The model under review builds one solid part; all positions refer to its coordinate system, in mm. A direction names the side the tool comes from. Round coordinates to 2 decimals unless told otherwise and drop trailing zeros. Write each loop counter-clockwise with the first axis right and the second up, starting at its lowest first coordinate (ties: lowest second). Pieces come first, ordered by that corner, then holes. Notation, with made-up numbers: (3, 15.5) - (27, 15.5) arc R7 ccw to (27, 21.5) - close; hole circle Ø5 at (76.5, 86). An arc over 180 degrees is marked (long way). One line per question, with ' | ' between items. Start each with the question number.
```python
from build123d import *

# Parameters (mm, degrees)
SKETCH1_W           = 183
SKETCH1_H           = 80.5
SKETCH1_W_2         = 163
SKETCH1_H_2         = 23
SKETCH1_R           = 1.6
BOSS_EXTRUDE1_DEPTH = 3.2
SKETCH1_3_W         = 183
SKETCH1_3_H         = 80.5
SKETCH1_3_R         = 1.6
SKETCH1_3_W_2       = 163
SKETCH1_3_H_2       = 23
BOSS_EXTRUDE2_DEPTH = 3


with BuildPart() as part:
    # Sketch1 → Boss-Extrude1 (new body)
    with BuildSketch(Plane(origin=(0, 0, 0), x_dir=(1, 0, 0), z_dir=(0, 1, 0))):
        Rectangle(SKETCH1_W, SKETCH1_H)
        with Locations((0, 17.25)):
            Rectangle(SKETCH1_W_2, SKETCH1_H_2, mode=Mode.SUBTRACT)
        Polygon((83.5, 2.75), (83.5, -2.75), (81.5, -2.75), (-81.5, -2.75), (-83.5, -2.75), (-83.5, 2.75), align=None, mode=Mode.SUBTRACT)
        with Locations((0, -17.25)):
            Rectangle(SKETCH1_W_2, SKETCH1_H_2, mode=Mode.SUBTRACT)
        Polygon((83.5, -31.75), (83.5, -37.25), (-81.5, -37.25), (-83.5, -37.25), (-83.5, -31.75), align=None, mode=Mode.SUBTRACT)
        Polygon((81.5, 37.25), (83.5, 37.25), (83.5, 31.75), (-83.5, 31.75), (-83.5, 37.25), align=None, mode=Mode.SUBTRACT)
        with Locations((-87.5, -34.5)):
            Circle(SKETCH1_R, mode=Mode.SUBTRACT)
        with Locations((-87.5, 0)):
            Circle(SKETCH1_R, mode=Mode.SUBTRACT)
        with Locations((-87.5, 34.5)):
            Circle(SKETCH1_R, mode=Mode.SUBTRACT)
        with Locations((87.5, 34.5)):
            Circle(SKETCH1_R, mode=Mode.SUBTRACT)
        with Locations((87.5, -34.5)):
            Circle(SKETCH1_R, mode=Mode.SUBTRACT)
        with Locations((87.5, 0)):
            Circle(SKETCH1_R, mode=Mode.SUBTRACT)
    extrude(amount=BOSS_EXTRUDE1_DEPTH)

    # Sketch1<3> → Boss-Extrude2 (add)
    with BuildSketch(Plane(origin=(0, 0, 0), x_dir=(1, 0, 0), z_dir=(0, 1, 0))):
        Rectangle(SKETCH1_3_W, SKETCH1_3_H)
        with Locations((-87.5, -34.5)):
            Circle(SKETCH1_3_R, mode=Mode.SUBTRACT)
        with Locations((0, -17.25)):
            Rectangle(SKETCH1_3_W_2, SKETCH1_3_H_2, mode=Mode.SUBTRACT)
        with Locations((87.5, -34.5)):
            Circle(SKETCH1_3_R, mode=Mode.SUBTRACT)
        with Locations((-87.5, 0)):
            Circle(SKETCH1_3_R, mode=Mode.SUBTRACT)
        with Locations((0, 17.25)):
            Rectangle(SKETCH1_3_W_2, SKETCH1_3_H_2, mode=Mode.SUBTRACT)
        with Locations((-87.5, 34.5)):
            Circle(SKETCH1_3_R, mode=Mode.SUBTRACT)
        with Locations((87.5, 0)):
            Circle(SKETCH1_3_R, mode=Mode.SUBTRACT)
        with Locations((87.5, 34.5)):
            Circle(SKETCH1_3_R, mode=Mode.SUBTRACT)
    extrude(amount=-BOSS_EXTRUDE2_DEPTH)


solid = part.part
```
1. Machinability: for faces 3 (the face through (-1, 0, 40.25)), 4 (the face through (-81.5, 0, 17)), 5 (the face through (83.5, 2, -35)), which of the approach directions +Z, -Z, +X, -X, +Y, -Y give a long, thin tool a straight path to every point of the face, cutting with its end or side? Answer none if there is none.
2. Add section A-A, the plane z = 20. Write out the cut boundary in (x, y), then the cut area to 3 significant figures.
3. Add section C-C, the plane x = 8. Write out the cut boundary in (y, z), then the cut area to 3 significant figures.
4. The part is to be moulded in two halves that separate along X. For faces 1 (the face through (-22, -3, -1)), 2 (the face through (-1, 0, -5.75)), say which applies: pulls with the +X half, pulls with the -X half, needs draft (parallel to the pull), parting line crosses it, or undercut.
5. Wall thickness on line 1 along Z through (x, y) = (-87.5, -0.75); line 2 along X through (y, z) = (0.5, 0); line 3 along Z through (x, y) = (-42.5, 0.5): over which ranges is each line inside the solid? List them lowest first. Write a range as [from, to].
6. Add section B-B, the plane y = -1.75. State how many separate pieces and enclosed holes the cut face has, then the cut area to 3 significant figures.
Geometry check:
1) face 3: +Z, +X, -X, +Y, -Y | face 4: +Y, -Y | face 5: +Y
2) outline: (-91.5, -3) - (-81.5, -3) - (-81.5, 3.2) - (-91.5, 3.2) - close; (81.5, -3) - (91.5, -3) - (91.5, 3.2) - (81.5, 3.2) - close | area: 124 mm2
3) outline: (-3, -40.25) - (3.2, -40.25) - (3.2, -37.25) - (0, -37.25) - (0, -31.75) - (3.2, -31.75) - (3.2, -28.75) - (-3, -28.75) - close; (-3, -5.75) - (3.2, -5.75) - (3.2, -2.75) - (0, -2.75) - (0, 2.75) - (3.2, 2.75) - (3.2, 5.75) - (-3, 5.75) - close; (-3, 28.75) - (3.2, 28.75) - (3.2, 31.75) - (0, 31.75) - (0, 37.25) - (3.2, 37.25) - (3.2, 40.25) - (-3, 40.25) - close | area: 161 mm2
4) face 1: needs draft | face 2: undercut
5) line 1: z = [-40.25, -36.1], [-32.9, -1.6], [1.6, 32.9], [36.1, 40.25] | line 2: x = [-91.5, -89.1], [-85.9, -83.5], [83.5, 85.9], [89.1, 91.5] | line 3: z = [-40.25, -37.25], [-31.75, -28.75], [-5.75, -2.75], [2.75, 5.75], [28.75, 31.75], [37.25, 40.25]
6) separate pieces: 1 | enclosed holes: 8 | area: 7,190 mm2
